Model file for the job. Use its own axes, mm. A direction names the side the tool comes from. Round coordinates to 2 decimals unless told otherwise and drop trailing zeros. Loops run counter-clockwise (first coordinate to the right, second up) from the corner with the lowest first, then second, coordinate; pieces in that order, holes last. Notation, with made-up numbers: M 63,14.5 L 102,14.5 A29 cw 102,51.5 Z; hole C -27,33 d6. An arc over 180 degrees is marked long. Answer in a Markdown table with one row per item.
from build123d import *

# Parameters (mm, degrees)
SKETCH_1_W               = 15
SKETCH_1_H               = 15
EXTRUDE_1_DEPTH          = 30
SKETCH_2_W               = 7
SKETCH_2_H               = 7
CUT_EXTRUDE_1_DEPTH      = 25
CUT_EXTRUDE_1_DEPTH_BACK = 0.001
FILLET_1_R               = 2


with BuildPart() as part:
    # 草图1 → 凸台-拉伸1 (new body)
    with BuildSketch(Plane.XY):
        Rectangle(SKETCH_1_W, SKETCH_1_H)
    extrude(amount=EXTRUDE_1_DEPTH)

    # 草图2 → 切除-拉伸1 (cut, two sides)
    with BuildSketch(Plane.XY) as cut_extrude_1_sk:
        Rectangle(SKETCH_2_W, SKETCH_2_H)
    extrude(amount=CUT_EXTRUDE_1_DEPTH, mode=Mode.SUBTRACT)
    extrude(cut_extrude_1_sk.sketch, amount=-CUT_EXTRUDE_1_DEPTH_BACK, mode=Mode.SUBTRACT)

    # 圆角1
    fillet_1_edges = [part.edges().sort_by_distance(p)[0] for p in [
        (-7.5, 0, 30),
        (0, -7.5, 30),
        (7.5, 0, 30),
        (0, 7.5, 30),
        (7.5, -7.5, 15),
        (-7.5, -7.5, 15),
        (-7.5, 7.5, 15),
        (7.5, 7.5, 15),
    ]]
    fillet(fillet_1_edges, radius=FILLET_1_R)


solid = part.part
1. Tool access for faces 1 (the cylindrical face through (6.9, -6.93, 14.2)), 2 (the flat face through (0, -3.5, 12)): list every direction of +Z, -Z, +X, -X, +Y, -Y with a clear straight run to the whole face (end or side of a thin tool).
Verdict:
| item | result |
|---|---|
| face 1 | +Z, -Z, +X, -Y |
| face 2 | -Z |
2. Mould opens along X. For faces 3 (the flat face through (0, 3.5, 12)), 4 (the flat face through (0, 5, 0)), 5 (the cylindrical face through (6.9, 0.08, 29.43)), 6 (the flat face through (-3.5, 0, 12)) say: +X half, -X half, draft (parallel to the pull), parting line (faces both ways), or undercut.
Verdict:
| item | result |
|---|---|
| face 3 | undercut |
| face 4 | draft |
| face 5 | +X half |
| face 6 | undercut |
3. Saw through at C-C (z = 25.5). Write the cut outline in (x, y).
Verdict:
| item | result |
|---|---|
| outline | M -7.5,-5.5 A2 ccw -5.5,-7.5 L 5.5,-7.5 A2 ccw 7.5,-5.5 L 7.5,5.5 A2 ccw 5.5,7.5 L -5.5,7.5 A2 ccw -7.5,5.5 Z |
4. Saw through at A-A (z = 11.25). Write the cut outline in (x, y).
Verdict:
| item | result |
|---|---|
| outline | M -7.5,-5.5 A2 ccw -5.5,-7.5 L 5.5,-7.5 A2 ccw 7.5,-5.5 L 7.5,5.5 A2 ccw 5.5,7.5 L -5.5,7.5 A2 ccw -7.5,5.5 Z; hole M -3.5,-3.5 L 3.5,-3.5 L 3.5,3.5 L -3.5,3.5 Z |
5. Saw through at B-B (x = -3). Write the cut outline in (y, z), and give its area (3 significant figures).
Verdict:
| item | result |
|---|---|
| outline | M -7.5,0 L -3.5,0 L -3.5,25 L 3.5,25 L 3.5,0 L 7.5,0 L 7.5,28 A2 ccw 5.5,30 L -5.5,30 A2 ccw -7.5,28 Z |
| area | 273 mm² |
6. Wall check: probe 1 along Y at (x, z) = (-1, 21.75); probe 2 along Z at (x, y) = (3, 0.25). Give the ranges that are in metal, low to high.
Verdict:
| item | result |
|---|---|
| probe 1 | y = -7.5 to -3.5, 3.5 to 7.5 |
| probe 2 | z = 25 to 30 |
7. Pin check, flat tip, straight feed: pin 1 (5.5 mm diameter, centred on x = 0, y = -0.5, fed in from -Z). Stop position of the tip, or through.
Verdict:
| item | result |
|---|---|
| pin 1 | stops at z = 25 |
